Work out the finished part from the listing and answer in its coordinate system (mm). A direction names the side the tool comes from. Coordinates: 2 decimals unless noted, no trailing zeros. Loops run counter-clockwise (first coordinate to the right, second up) from the corner with the lowest first, then second, coordinate; pieces in that order, holes last. Notation, with made-up numbers: (11, 43) - (16, 43) arc R22 cw to (16, 76) - close; hole circle Ø9 at (37, 6.25). An arc over 180 degrees is marked (long way). Write each question's results on one line, items separated by ' | '. Start each with the question number.
Item 1: Each of these flat-tipped pins is pushed along its axis until it touches: pin 1 Ø1 at (y, z) = (-9, 1) entering from +X; pin 2 Ø1.6 at (y, z) = (-3.5, 1.5) entering from -X. Where does it stop, or does it pass through?
Item 2: Section C-C, the plane z = 0.85 is taken. Write down the section's boundary in (x, y), plus the area to 3 significant figures.
Item 3: Consider probe 1 along X at (y, z) = (-5.5, 0.75); probe 2 along Y at (x, z) = (73.5, 2.1); probe 3 along Y at (x, z) = (23.5, 1.1). Determine where each line is inside the solid, lowest interval first. Write a range as [from, to].
Item 4: A tool of negligible diameter and unlimited length cuts with its end or side. For faces 1 (the face through (70, -6, 2)), 2 (the face through (10, 0, 2)), 3 (the face through (79, 13, 0)), from which of +Z, -Z, +X, -X, +Y, -Y can it reach the whole face along a straight path? Write none if from no direction.
from build123d import *

# Parameters (mm, degrees)
BOSS_EXTRUDE1_DEPTH = 3.175
CHAMFER1_SIZE       = 1.5875


with BuildPart() as part:
    # Sketch1 → Boss-Extrude1 (new body)
    with BuildSketch(Plane.XY):
        Polygon((0, 0), (20, 0), (20, -12.75), (70, -12.75), (70, 0), (130, 0), (115, 55), (100, 55), align=None)
    extrude(amount=BOSS_EXTRUDE1_DEPTH)

    # Chamfer1
    chamfer1_edges = [part.edges().sort_by_distance(p)[0] for p in [
        (50, 27.5, 3.175),
        (107.5, 55, 3.175),
        (122.5, 27.5, 3.175),
        (50, 27.5, 0),
        (107.5, 55, 0),
        (122.5, 27.5, 0),
    ]]
    chamfer(chamfer1_edges, length=CHAMFER1_SIZE - 0.0001)  # a hair under: the kernel refuses the full size


solid = part.part
Answer key:
1) pin 1: stops at x = 70 | pin 2: stops at x = 20
2) outline: (1.53, 0) - (20, 0) - (20, -12.75) - (70, -12.75) - (70, 0) - (129.24, 0) - (114.44, 54.26) - (100.19, 54.26) - close | area: 4,490 mm^2
3) probe 1: x = [20, 70] | probe 2: y = [0, 39.84] | probe 3: y = [-12.75, 12.37]
4) face 1: +Z, -Z, +X, -Y | face 2: +Z, -Z, -X, -Y | face 3: -Z, +X, -X, +Y, -Y
